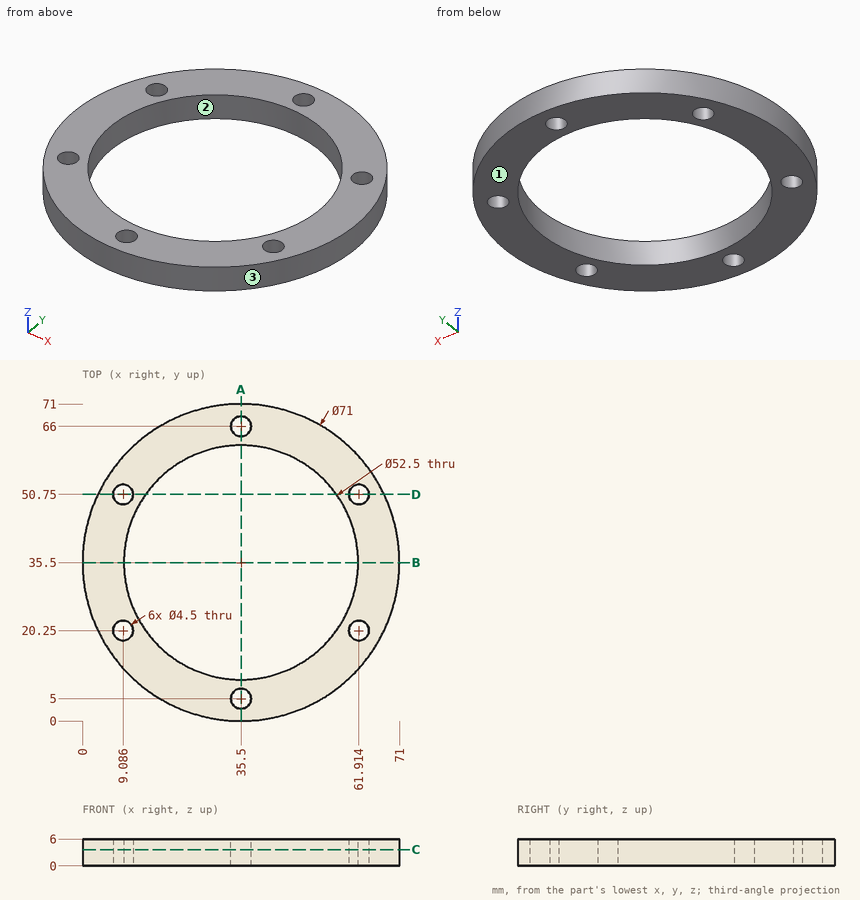
Print and shaded views of the part. All mm, measured from the part's lowest x, y and z. Round coordinates to 2 decimals unless told otherwise and drop trailing zeros. Write each loop counter-clockwise with the first axis right and the second up, starting at its lowest first coordinate (ties: lowest second). Pieces come first, ordered by that corner, then holes.
Item 1: Cut at C-C, the plane z = 3.6. Give the cut face in (x, y), plus the area to 3 significant figures.
Results:
outline: circle Ø71 at (35.5, 35.5); hole circle Ø4.5 at (9.09, 20.25); hole circle Ø4.5 at (9.09, 50.75); hole circle Ø52.5 at (35.5, 35.5); hole circle Ø4.5 at (35.5, 5); hole circle Ø4.5 at (35.5, 66); hole circle Ø4.5 at (61.91, 20.25); hole circle Ø4.5 at (61.91, 50.75)
area: 1,700 mm2
Item 2: Probe L1, parallel to Y at x = 35.5, z = 3.05; L2, parallel to X at y = 49, z = 4.95; L3, parallel to Y at x = 14, z = 2.4. List the from-to ranges inside material, lowest first.
Results:
L1: y = 0 to 2.75, 7.25 to 9.25, 61.75 to 63.75, 68.25 to 71
L2: x = 2.67 to 7.67, 10.5 to 12.99, 58.01 to 60.5, 63.33 to 68.33
L3: y = 7.25 to 20.44, 50.56 to 63.75
Item 3: Cut at D-D, the plane y = 50.75. Give the cut face in (x, z), plus the area to 3 significant figures.
Results:
outline: (3.44, 0) - (6.84, 0) - (6.84, 6) - (3.44, 6) - close; (11.34, 0) - (14.13, 0) - (14.13, 6) - (11.34, 6) - close; (56.87, 0) - (59.66, 0) - (59.66, 6) - (56.87, 6) - close; (64.16, 0) - (67.56, 0) - (67.56, 6) - (64.16, 6) - close
area: 74.3 mm2
Item 4: Two-plate mould, pull along X, no slides. Class the marked faces 1, 2 and 3: +X half, -X half, draft (parallel to the pull), parting line (faces both ways), or undercut.
Results:
face 1: draft
face 2: undercut
face 3: parting line
Item 5: Cut at B-B, the plane y = 35.5. Give the cut face in (x, z).
Results:
outline: (0, 0) - (9.25, 0) - (9.25, 6) - (0, 6) - close; (61.75, 0) - (71, 0) - (71, 6) - (61.75, 6) - close
Item 6: Cut at A-A, the plane x = 35.5. Give the cut face in (y, z), plus the area to 3 significant figures.
Results:
outline: (0, 0) - (2.75, 0) - (2.75, 6) - (0, 6) - close; (7.25, 0) - (9.25, 0) - (9.25, 6) - (7.25, 6) - close; (61.75, 0) - (63.75, 0) - (63.75, 6) - (61.75, 6) - close; (68.25, 0) - (71, 0) - (71, 6) - (68.25, 6) - close
area: 57.0 mm2
Item 7: Drop flat-ended pins along their axis: pin 1 Ø3 at (x, z) = (21.5, 2.5) entering from +Y; pin 2 Ø2 at (x, z) = (38, 2.5) entering from -Y. Give the stop position or say it passes through.
Results:
pin 1: stops at y = 68.73
pin 2: stops at y = 0.03
